```python
from build123d import *

# Parameters (mm, degrees)
SKETCH1_R                 = 9.525
SKETCH1_R_2               = 2
BOSS_EXTRUDE1_DEPTH       = 5.08
F_4_40_TAPPED_HOLE3_D     = 2.2606
F_4_40_TAPPED_HOLE3_DEPTH = 7.6
F_4_40_TAPPED_HOLE3_TIP   = 0.679152758
F_4_40_TAPPED_HOLE2_D     = 2.2606
F_4_40_TAPPED_HOLE2_DEPTH = 7.6
F_4_40_TAPPED_HOLE2_TIP   = 0.679152758


with BuildPart() as part:
    # Sketch1 → Boss-Extrude1 (new body)
    with BuildSketch(Plane.XY):
        Circle(SKETCH1_R)
        Circle(SKETCH1_R_2, mode=Mode.SUBTRACT)
    extrude(amount=BOSS_EXTRUDE1_DEPTH)

    # #4-40 Tapped Hole3
    with Locations(Plane.XY.offset(5.08)):
        with Locations((-6.35, 0), (6.35, 0), (0, 6.35), (0, -6.35)):
            Hole(F_4_40_TAPPED_HOLE3_D / 2, depth=F_4_40_TAPPED_HOLE3_DEPTH)
            with Locations((0, 0, -(F_4_40_TAPPED_HOLE3_DEPTH + F_4_40_TAPPED_HOLE3_TIP / 2))):  # 118° drill point
                Cone(0, F_4_40_TAPPED_HOLE3_D / 2, F_4_40_TAPPED_HOLE3_TIP, mode=Mode.SUBTRACT)

    # #4-40 Tapped Hole2
    with Locations(Plane(origin=(6.681738172, 6.788225099, 2.54), x_dir=(0.712674551117, -0.701494821214, 0), z_dir=(0.701494821214, 0.712674551117, 0))):
        with Locations((0, 0)):
            Hole(F_4_40_TAPPED_HOLE2_D / 2, depth=F_4_40_TAPPED_HOLE2_DEPTH)
            with Locations((0, 0, -(F_4_40_TAPPED_HOLE2_DEPTH + F_4_40_TAPPED_HOLE2_TIP / 2))):  # 118° drill point
                Cone(0, F_4_40_TAPPED_HOLE2_D / 2, F_4_40_TAPPED_HOLE2_TIP, mode=Mode.SUBTRACT)


solid = part.part
```
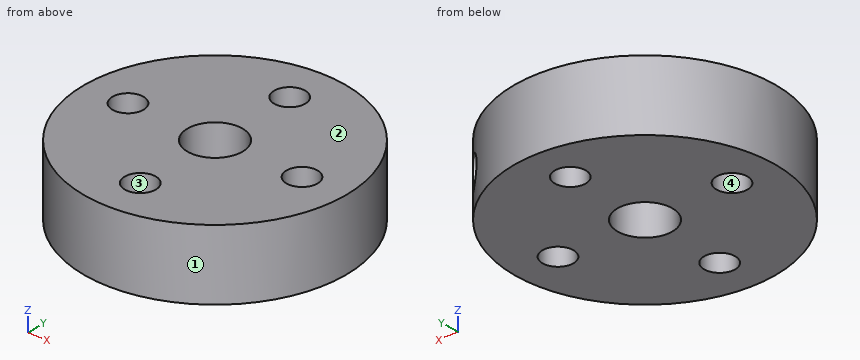
The model under review builds one solid part; all positions refer to its coordinate system, in mm. Face numbers are marked on the shaded views. Give positions to 0.01 mm unless a question says otherwise; leave off trailing zeros. Write each loop counter-clockwise with the first axis right and the second up, starting at its lowest first coordinate (ties: lowest second). Pieces come first, ordered by that corner, then holes. Notation, with made-up numbers: M 77,46 L 120,46 A27 cw 120,82 Z; hole C 9.25,-1 d11. An arc over 180 degrees is marked long. Write item = value, one per line. Start each with the question number.
Q1. Mouldability with a two-part tool opening along X and no side actions: class the marked faces 1, 2, 3 and 4 as released by +X, released by -X, zero draft, split by the parting line, or undercut.
Q2. We need section A-A (x = 0). State the section outline as (y, z) points (3 decimals), plus the area to 3 significant figures.
Q3. For line 1 (Y direction, x = 0, z = 3.85) (3 decimals); line 2 (Y direction, x = 5.5, z = 2.4); line 3 (X direction, y = 6.5, z = 4.05), list the stretches that pass through material, from the lowest coordinate up.
Q4. We need section C-C (y = -6.35). State the section outline as (x, z) points, plus the area to 3 significant figures.
Q5. We need section B-B (z = 1.1). State the section outline as (x, y) points (3 decimals).
Q6. Clearance check with flat-ended pins moving along their axes: pin 1 (1 mm diameter, centred on x = -4, z = 3, fed in from -Y); pin 2 (3 mm diameter, centred on x = 4.5, z = 2, fed in from -Y). State where each tip first meets the part, or that it passes through.
Result set:
q1.face_1 = split by the parting line
q1.face_2 = zero draft
q1.face_3 = undercut
q1.face_4 = undercut
q2.outline = M -9.525,0 L -7.48,0 L -7.48,5.08 L -9.525,5.08 Z; M -5.22,0 L -2,0 L -2,5.08 L -5.22,5.08 Z; M 2,0 L 5.22,0 L 5.22,5.08 L 2,5.08 Z; M 7.48,0 L 9.525,0 L 9.525,5.08 L 7.48,5.08 Z
q2.area = 53.5 mm2
q3.line_1 = -9.525 to -7.48, -5.22 to -2, 2 to 5.22, 7.48 to 9.525
q3.line_2 = -7.78 to -0.75, 0.75 to 3.99, 7.19 to 7.78
q3.line_3 = -6.96 to -1.12, 1.12 to 6.96
q4.outline = M -7.1,0 L -1.13,0 L -1.13,5.08 L -7.1,5.08 Z; M 1.13,0 L 7.1,0 L 7.1,5.08 L 1.13,5.08 Z
q4.area = 60.6 mm2
q5.outline = C 0,0 d19.05; hole C -6.35,0 d2.261; hole C 0,0 d4; hole C 0,-6.35 d2.261; hole C 0,6.35 d2.261; hole C 6.35,0 d2.261
q6.pin_1 = -8.86
q6.pin_2 = -9.04
